Source: three-view drawing plus pictorial views. Frame: mm from the lowest corner of the part. A direction names the side the tool comes from. Give positions to 0.01 mm unless a question says otherwise; leave off trailing zeros. Loops run counter-clockwise (first coordinate to the right, second up) from the corner with the lowest first, then second, coordinate; pieces in that order, holes last. Notation, with made-up numbers: M 7,-25 L 53,-25 A22 cw 53,-12 Z; hole C 57.5,65.25 d5. An arc over 180 degrees is marked long. One line per item, written item: value. Start each with the question number.
(1) Access query for the marked faces 4 and 5. Directions: +Z, -Z, +X, -X, +Y, -Y. A direction counts if a zero-diameter tool reaches every point of the face in a straight line with its end or side. Return the directions, or none.
(2) Pin query (flat end, axial travel): P1, Ø2, axis at y = 8, z = 3, coming from the -X side; P2, Ø3, axis at x = 71, z = 10, coming from the +Y side; P3, Ø3, axis at x = 70.5, z = 8, coming from the -Y side; P4, Ø3, axis at x = 4, z = 12, coming from the -Y side. Return the tip coordinate at first contact, or that it passes through.
(3) Ray query, line 1 along X through (y, z) = (4, 9); line 2 along X through (y, z) = (3, 1.25); line 3 along Z through (x, y) = (23, 2). Return the intervals inside material, ascending. Write a range as from..to.
(4) Section A-A on z = 14.25. Output: boundary loops of the cut face in (x, y).
(5) Pull-direction query (X, two-part tool) for the marked faces 1, 2 and 3; classes: released by +X, released by -X, zero draft, split by the parting line, or undercut.
(6) Section C-C on y = 7.25. Output: boundary loops of the cut face in (x, z).
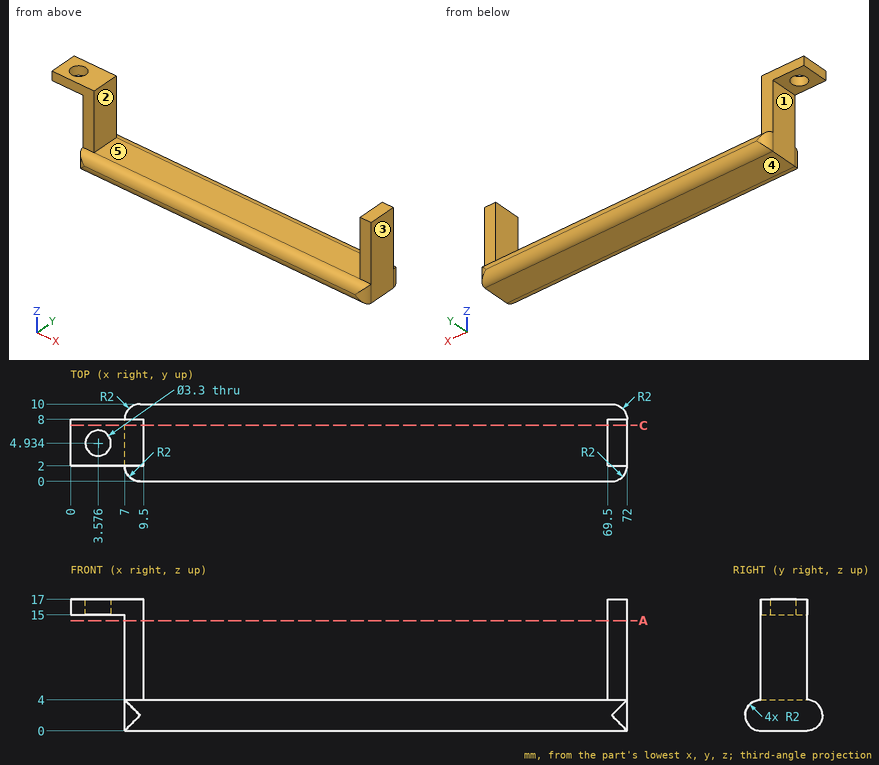
Output values:
1. face 4: -Z, +X, -X, +Y, -Y
1. face 5: +Z, +Y, -Y
2. P1: stops at x = 7
2. P2: stops at y = 8
2. P3: stops at y = 2
2. P4: passes through
3. line 1: x = 7..9.5, 69.5..72
3. line 2: x = 7..72
3. line 3: z = 0..4
4. outline: M 7,2 L 9.5,2 L 9.5,8 L 7,8 Z; M 69.5,2 L 72,2 L 72,8 L 69.5,8 Z
5. face 1: released by -X
5. face 2: undercut
5. face 3: released by +X
6. outline: M 0,15 L 7,15 L 7,0 L 72,0 L 72,17 L 69.5,17 L 69.5,4 L 9.5,4 L 9.5,17 L 0,17 Z
